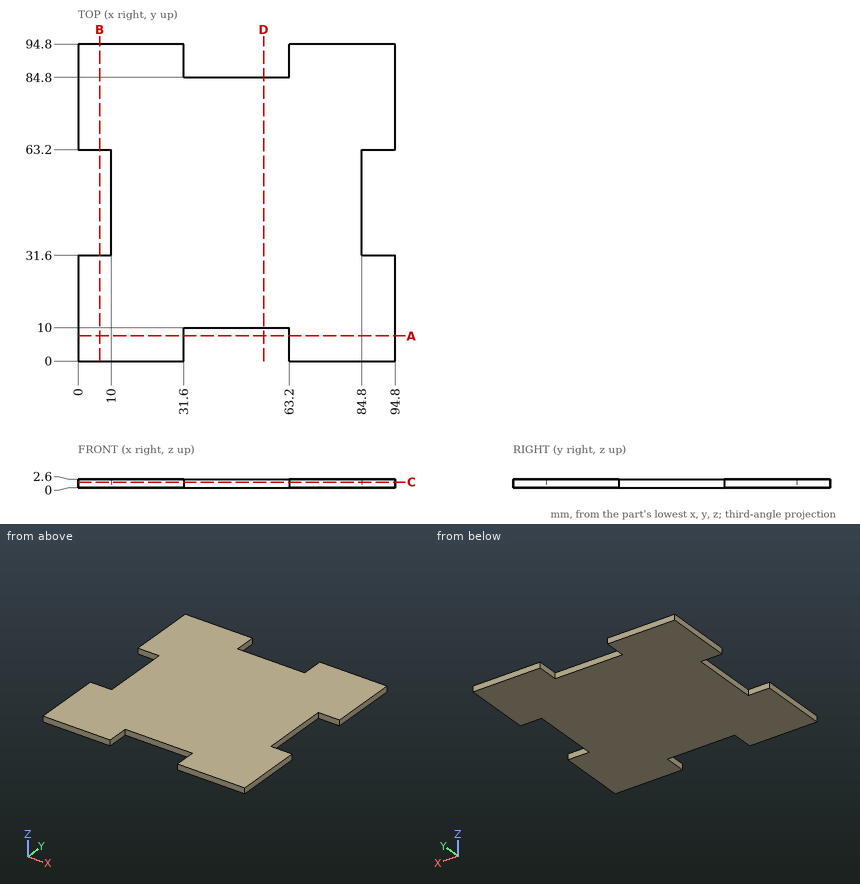
For this review, use the dimensioned drawing (mm, ordinates from the lowest corner) and the shaded views. Give positions to 0.01 mm unless a question says otherwise; leave off trailing zeros. Order: outer loops, then holes, each group sorted by start corner. A loop starts at its lowest first (then second) coordinate and runs counter-clockwise, first axis right, second up.
1) Insertion check: pin 1 (1.3 mm diameter, centred on y = 43.5, z = 1, fed in from +X); pin 2 (1 mm diameter, centred on x = 38, z = 1.5, fed in from +Y); pin 3 (0.8 mm diameter, centred on y = 40, z = 1.5, fed in from -X). Each pin has a flat end and moves straight along its axis. Give the tip position at first contact, or say it passes through.
2) Take a section at C-C (z = 1.7). Give the boundary of the cut face in (x, y).
3) Take a section at D-D (x = 55.5). Give the boundary of the cut face in (y, z).
4) Wall thickness on line 1 (X direction, y = 8.5, z = 1.85); line 2 (X direction, y = 53, z = 0.2): over which ranges is each line inside the solid? List them lowest first.
5) Take a section at A-A (y = 7.5). Give the boundary of the cut face in (x, z), then the cut area to 3 significant figures.
Derived:
1. pin 1: stops at x = 84.8
1. pin 2: stops at y = 84.8
1. pin 3: stops at x = 10
2. outline: (0, 0) - (31.6, 0) - (31.6, 10) - (63.2, 10) - (63.2, 0) - (94.8, 0) - (94.8, 31.6) - (84.8, 31.6) - (84.8, 63.2) - (94.8, 63.2) - (94.8, 94.8) - (63.2, 94.8) - (63.2, 84.8) - (31.6, 84.8) - (31.6, 94.8) - (0, 94.8) - (0, 63.2) - (10, 63.2) - (10, 31.6) - (0, 31.6) - close
3. outline: (10, 0) - (84.8, 0) - (84.8, 2.6) - (10, 2.6) - close
4. line 1: x = 0 to 31.6, 63.2 to 94.8
4. line 2: x = 10 to 84.8
5. outline: (0, 0) - (31.6, 0) - (31.6, 2.6) - (0, 2.6) - close; (63.2, 0) - (94.8, 0) - (94.8, 2.6) - (63.2, 2.6) - close
5. area: 164 mm2
